Verification items for the finished model (mm, model axes). A direction names the side the tool comes from. Coordinates: 2 decimals unless noted, no trailing zeros. Write each loop counter-clockwise with the first axis right and the second up, starting at its lowest first coordinate (ties: lowest second). Pieces come first, ordered by that corner, then holes. Notation, with made-up numbers: (-8, -6.75) -> (45, -6.75) arc R23 ccw to (45, 5.25) -> close; hole circle Ø5 at (79.5, -25.5). An arc over 180 degrees is marked (long way). Answer in a Markdown table with one row per item.
```python
from build123d import *

# Parameters (mm, degrees)
F0_W     = 10
F0_H     = 10
F1_DEPTH = 10
F2_R     = 1.35
F3_DEPTH = 5.15
F4_R     = 0.5
F5_DEPTH = 10.001


with BuildPart() as f1:
    # F0 (on Top) → F1 (new body)
    with BuildSketch(Plane.XY):
        with Locations((5, 5)):
            Rectangle(F0_W, F0_H)
    extrude(amount=F1_DEPTH)

    # F2 (on face) → F3 (cut)
    with BuildSketch(Plane.XY.offset(10)):
        with Locations((5, 5)):
            Circle(F2_R)
    extrude(amount=-F3_DEPTH, mode=Mode.SUBTRACT)

    # F4 (on face) → F5 (cut, through all)
    with BuildSketch(Plane.XZ):
        with Locations((0.903822, 8.507882)):
            Circle(F4_R)
    extrude(amount=-F5_DEPTH, mode=Mode.SUBTRACT)


solid = f1.part
```
1. Tool access check on faces 1 (the flat face through (0, 5, 5)), 2 (the cylindrical face through (6.288, 5.406, 7.461)). Record the directions out of +Z, -Z, +X, -X, +Y, -Y that give a thin tool (end or side, any length) a straight path to the whole face; none if there is none.
Geometry says:
| item | result |
|---|---|
| face 1 | +Z, -Z, -X, +Y, -Y |
| face 2 | +Z |
2. Thickness scan on line 1 (X direction, y = 3, z = 8.5); line 2 (Y direction, x = 5, z = 6); line 3 (Z direction, x = 1, y = 8.25). Record the ranges inside material, lowest first. Write a range as from..to.
Geometry says:
| item | result |
|---|---|
| line 1 | 0..0.4, 1.4..10 |
| line 2 | 0..3.65, 6.35..10 |
| line 3 | 0..8.02, 9..10 |
3. Section check D-D, the plane x = 0.75. Record the boundary of the cut face in (y, z), plus the area to 3 significant figures.
Geometry says:
| item | result |
|---|---|
| outline | (0, 0) -> (10, 0) -> (10, 8.03) -> (0, 8.03) -> close; (0, 8.98) -> (10, 8.98) -> (10, 10) -> (0, 10) -> close |
| area | 90.5 mm^2 |
4. Section check B-B, the plane x = 5. Record the boundary of the cut face in (y, z), plus the area to 3 significant figures.
Geometry says:
| item | result |
|---|---|
| outline | (0, 0) -> (10, 0) -> (10, 10) -> (6.35, 10) -> (6.35, 4.85) -> (3.65, 4.85) -> (3.65, 10) -> (0, 10) -> close |
| area | 86.1 mm^2 |
5. Section check C-C, the plane y = 6. Record the boundary of the cut face in (x, z).
Geometry says:
| item | result |
|---|---|
| outline | (0, 0) -> (10, 0) -> (10, 10) -> (5.91, 10) -> (5.91, 4.85) -> (4.09, 4.85) -> (4.09, 10) -> (0, 10) -> close; hole circle Ø1 at (0.9, 8.51) |
6. Mould release check, pull along Z, two halves, no side actions. Record for faces 3 (the flat face through (6, 6.2, 10)), 4 (the flat face through (5, 5, 0)), 5 (the flat face through (5, 10, 5)), 6 (the cylindrical face through (0.51, 4.93, 8.2)): released by +Z, released by -Z, zero draft, split by the parting line, or undercut.
Geometry says:
| item | result |
|---|---|
| face 3 | released by +Z |
| face 4 | released by -Z |
| face 5 | zero draft |
| face 6 | undercut |
7. Depth check by flat-ended pin: P1, Ø2.5, axis at x = 5, y = 5, coming from the +Z side. Enter the tip coordinate at first touch or a pass-through.
Geometry says:
| item | result |
|---|---|
| P1 | z = 4.85 |
8. Section check A-A, the plane z = 8.75. Record the boundary of the cut face in (x, y), plus the area to 3 significant figures.
Geometry says:
| item | result |
|---|---|
| outline | (0, 0) -> (0.47, 0) -> (0.47, 10) -> (0, 10) -> close; (1.34, 0) -> (10, 0) -> (10, 10) -> (1.34, 10) -> close; hole circle Ø2.7 at (5, 5) |
| area | 85.5 mm^2 |
